The model under review builds one solid part; all positions refer to its coordinate system, in mm. Face numbers are marked on the shaded views. Round coordinates to 2 decimals unless told otherwise and drop trailing zeros. Write each loop counter-clockwise with the first axis right and the second up, starting at its lowest first coordinate (ties: lowest second). Pieces come first, ordered by that corner, then holes. Notation, with made-up numbers: (-34, 32.5) - (-23, 32.5) arc R27 cw to (-23, 58.5) - close; hole circle Ø4 at (76, -8.5). An arc over 180 degrees is marked (long way). Use one line per item in the form item = value.
Autodesk Inventor part; units mm, degrees
ref_plane "YZ Plane" through (0, 0, 0) normal (1, 0, 0) x (0, 1, 0)
ref_plane "XZ Plane" through (0, 0, 0) normal (0, 1, 0) x (-1, 0, 0)
ref_plane "XY Plane" through (0, 0, 0) normal (0, 0, 1) x (1, 0, 0)
sketch "Esquisse1" plane through (0, 0, 0) normal (0, 1, 0) x (-1, 0, 0)
  line L0 (-30, 27) -> (30, 27)
  line L1 (30, 27) -> (30, -27)
  line L2 (30, -27) -> (-30, -27)
  line L3 (-30, -27) -> (-30, 27)
  line L4 (-30, 27) -> (30, -27) construction
  line L5 (30, 27) -> (-30, -27) construction
  circle A0 centre (0, -7) radius 6.25
  point P0 (0, 0)
  dimension "d0" = 54
  dimension "d1" = 60
  dimension "d2" = 34
  dimension "d3" = 12.5
extrude "Extrusion1" add sketch "Esquisse1" along normal blind 14.5
sketch "Esquisse2" plane through (-30, 0, 27) normal (0, 0, 1) x (1, 0, 0)
  line L0 (0, 0) -> (0, 14.5)
  line L1 (60, 0) -> (0, 0)
  line L2 (0, 14.5) -> (60, 14.5)
  line L3 (60, 14.5) -> (60, 0)
  line L4 (60, 0) -> (0, 0)
  line L5 (0, 0) -> (0, 14.5)
  line L6 (0, 7.25) -> (60, 7.25)
  circle A0 centre (15, 7.25) radius 1.75
  circle A1 centre (45, 7.25) radius 1.75
  point P0 (30, 0)
  dimension "d6" = 15
  dimension "d7" = 15
  dimension "d8" = 3.5
fillet "Congé1" radius 1 9 edges at (-30, 14.5, 0) (0, 14.5, -27) (30, 14.5, 0) (0, 14.5, 27) (30, 7.25, 27) (-30, 7.25, 27) (-30, 7.25, -27) (30, 7.25, -27) (6.25, 14.5, -7)
extrude "Extrusion2" cut sketch "Esquisse2" against normal blind 10 contours A0 L6 | L6 A0 | A1 L6 | L6 A1
properties part number "dessus_cadre"
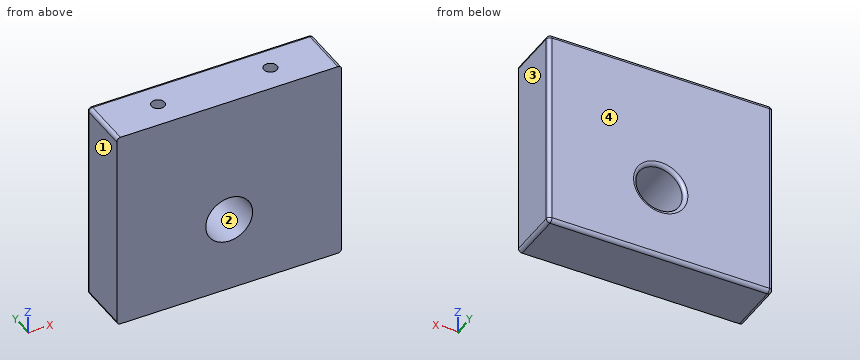
(1) Add section A-A on x = 0. Write out the cut boundary in (y, z), then the cut area to 3 significant figures.
Geometry results:
outline = (0, -27) - (13.5, -27) arc R1 ccw to (14.5, -26) - (14.5, -14.25) arc R1 ccw to (13.5, -13.25) - (0, -13.25) - close; (0, -0.75) - (13.5, -0.75) arc R1 ccw to (14.5, 0.25) - (14.5, 26) arc R1 ccw to (13.5, 27) - (0, 27) - close
area = 601 mm2
(2) Add section C-C on z = -7. Write out the cut boundary in (x, y), then the cut area to 3 significant figures.
Geometry results:
outline = (-30, 0) - (-6.25, 0) - (-6.25, 13.5) arc R1 ccw to (-7.25, 14.5) - (-29, 14.5) arc R1 ccw to (-30, 13.5) - close; (6.25, 0) - (30, 0) - (30, 13.5) arc R1 ccw to (29, 14.5) - (7.25, 14.5) arc R1 ccw to (6.25, 13.5) - close
area = 688 mm2
(3) The part is to be moulded in two halves that separate along X. For the marked faces 1, 2, 3 and 4, say which applies: +X half, -X half, draft (parallel to the pull), parting line (faces both ways), or undercut.
Geometry results:
face_1 = -X half
face_2 = undercut
face_3 = +X half
face_4 = draft
(4) Insertion check: P1, Ø1.8, axis at x = -14.5, y = 7.5, coming from the +Z side; P2, Ø11, axis at x = 0, z = -7, coming from the +Y side. Each pin has a flat end and moves straight along its axis. Give the tip position at first contact, or say it passes through.
Geometry results:
P1 = 17
P2 = through
(5) Add section B-B on y = 7.25. Write out the cut boundary in (x, z).
Geometry results:
outline = (-30, -26) arc R1 ccw to (-29, -27) - (29, -27) arc R1 ccw to (30, -26) - (30, 26) arc R1 ccw to (29, 27) - (16.75, 27) - (16.75, 17) - (13.25, 17) - (13.25, 27) - (-13.25, 27) - (-13.25, 17) - (-16.75, 17) - (-16.75, 27) - (-29, 27) arc R1 ccw to (-30, 26) - close; hole circle Ø12.5 at (0, -7)
(6) Add section D-D on x = -15. Write out the cut boundary in (y, z), then the cut area to 3 significant figures.
Geometry results:
outline = (0, -27) - (13.5, -27) arc R1 ccw to (14.5, -26) - (14.5, 26) arc R1 ccw to (13.5, 27) - (9, 27) - (9, 17) - (5.5, 17) - (5.5, 27) - (0, 27) - close
area = 748 mm2
(7) To check wall thickness, follow L1, parallel to X at y = 7.25, z = 21; L2, parallel to Z at x = 0, y = 6.75; L3, parallel to Y at x = -15, z = 20.75. State the ranges of each line that lie inside material, in increasing order.
Geometry results:
L1 = -30 to -16.75, -13.25 to 13.25, 16.75 to 30
L2 = -27 to -13.25, -0.75 to 27
L3 = 0 to 5.5, 9 to 14.5
